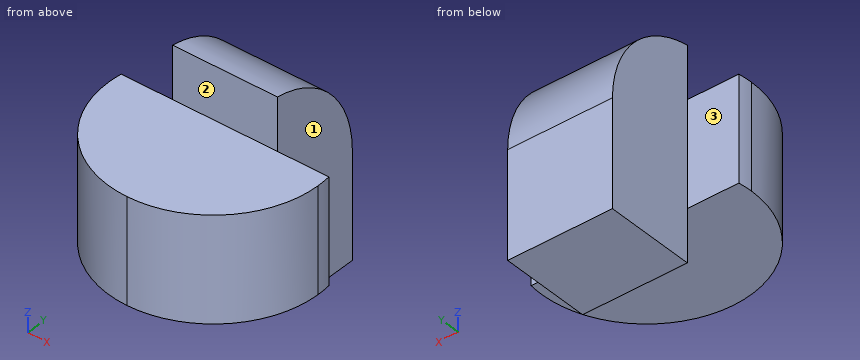
from build123d import *

# Parameters (mm, degrees)
SKETCH1_W           = 40
SKETCH1_H           = 40
BOSS_EXTRUDE1_DEPTH = 40
SKETCH2_W           = 10
SKETCH2_H           = 20
CUT_EXTRUDE1_DEPTH  = 40
SKETCH3_W           = 10
SKETCH3_H           = 10
CUT_EXTRUDE2_DEPTH  = 40
CUT_EXTRUDE3_DEPTH  = 40
SKETCH5_W           = 20
SKETCH5_H           = 10
CUT_EXTRUDE4_DEPTH  = 40
SKETCH6_W           = 20
SKETCH6_H           = 19.641016119
CUT_EXTRUDE5_DEPTH  = 40
BOSS_EXTRUDE2_DEPTH = 20


with BuildPart() as part:
    # Sketch1 → Boss-Extrude1 (new body)
    with BuildSketch(Plane.XY):
        with Locations((20, 20)):
            Rectangle(SKETCH1_W, SKETCH1_H)
    extrude(amount=BOSS_EXTRUDE1_DEPTH)

    # Sketch2 → Cut-Extrude1 (cut)
    with BuildSketch(Plane.XY.offset(40)):
        with BuildLine():
            ThreePointArc((20, 0), (5.857864376, 5.857864376), (0, 20))
            Line((0, 20), (0, 0))
            Line((0, 0), (20, 0))
        make_face()
        with BuildLine():
            ThreePointArc((40, 20), (34.142135624, 5.857864376), (20, 0))
            Line((20, 0), (40, 0))
            Line((40, 0), (40, 20))
        make_face()
        with Locations((35, 30)):
            Rectangle(SKETCH2_W, SKETCH2_H)
        with Locations((5, 30)):
            Rectangle(SKETCH2_W, SKETCH2_H)
    extrude(amount=-CUT_EXTRUDE1_DEPTH, mode=Mode.SUBTRACT)

    # Sketch3 → Cut-Extrude2 (cut)
    with BuildSketch(Plane(origin=(0, 20, 0), x_dir=(1, 0, 0), z_dir=(0, 1, 0))):
        with Locations((5, -5)):
            Rectangle(SKETCH3_W, SKETCH3_H)
        with Locations((35, -5)):
            Rectangle(SKETCH3_W, SKETCH3_H)
        with Locations((35, -35)):
            Rectangle(SKETCH3_W, SKETCH3_H)
        with Locations((5, -35)):
            Rectangle(SKETCH3_W, SKETCH3_H)
    extrude(amount=-CUT_EXTRUDE2_DEPTH, mode=Mode.SUBTRACT)

    # Sketch4 → Cut-Extrude3 (cut)
    with BuildSketch(Plane.ZY.offset(-10)):
        Polygon((10, 22.679491924), (0, 22.679491924), (0, 2.679491924), (10, 2.679491924), (10, 20), align=None)
        Polygon((30, 2.679491924), (40, 2.679491924), (40, 22.679491924), (30, 22.679491924), (30, 20), align=None)
        with BuildLine():
            ThreePointArc((20.358983897, 39.999201827), (33.408185604, 35.000772179), (40, 22.679491924))
            Line((40, 22.679491924), (40, 40))
            Line((40, 40), (20.358983897, 39.999201827))
        make_face()
    extrude(amount=-CUT_EXTRUDE3_DEPTH, mode=Mode.SUBTRACT)

    # Sketch5 → Cut-Extrude4 (cut)
    with BuildSketch(Plane(origin=(0, 2.679491924, 0), x_dir=(1, 0, 0), z_dir=(0, 1, 0))):
        with Locations((20, -5)):
            Rectangle(SKETCH5_W, SKETCH5_H)
        with Locations((20, -35)):
            Rectangle(SKETCH5_W, SKETCH5_H)
    extrude(amount=-CUT_EXTRUDE4_DEPTH, mode=Mode.SUBTRACT)

    # Sketch6 → Cut-Extrude5 (cut)
    with BuildSketch(Plane(origin=(0, 39.998374412, -0.001625456), x_dir=(1, 0, 0), z_dir=(0, -0.999999999, 4.0638e-05))):
        with Locations((20, 30.18111743)):
            Rectangle(SKETCH6_W, SKETCH6_H)
    extrude(amount=-CUT_EXTRUDE5_DEPTH, mode=Mode.SUBTRACT)

    # Sketch8 → Boss-Extrude2 (add)
    with BuildSketch(Plane.XY.offset(30)):
        with BuildLine():
            Line((0.180304669, 22.679491924), (39.819695331, 22.679491924))
            ThreePointArc((39.819695331, 22.679491924), (20, 0), (0.180304669, 22.679491924))
        make_face()
    extrude(amount=-BOSS_EXTRUDE2_DEPTH)


solid = part.part
Could you check a few things on this model? Use its own coordinates, in mm. Face numbers are marked on the shaded views. A direction names the side the tool comes from. Coordinates: 2 decimals unless noted, no trailing zeros. Order: outer loops, then holes, each group sorted by start corner. A loop starts at its lowest first (then second) coordinate and runs counter-clockwise, first axis right, second up. Notation, with made-up numbers: (37, 80) -> (44, 80) arc R18 cw to (44, 99) -> close; hole circle Ø1 at (-18.75, 68.5). An arc over 180 degrees is marked (long way). One line per question, with ' | ' between items.
Q1. I'm going to push flat-ended pins straight in: P1, Ø8.5, axis at y = 29.5, z = 11, coming from the +X side; P2, Ø2, axis at x = 16.5, z = 29, coming from the -Y side; P3, Ø3, axis at x = 25, z = 4, coming from the -Y side; P4, Ø6, axis at x = 4.5, z = 5, coming from the -Y side. Where does each tip first touch, or does it pass through?
Return value:
P1: x = 30 | P2: y = 0.16 | P3: y = 22.68 | P4: through
Q2. Imagine slicing it at C-C on y = 4. Please give me the cut outline in (x, z).
Return value:
outline: (8, 10) -> (32, 10) -> (32, 30) -> (8, 30) -> close
Q3. If I drill on L1, parallel to Z at x = 17, y = 17; L2, parallel to Y at x = 13, z = 9, over which ranges is the centre line in solid material (lowest first)?
Return value:
L1: 10 to 30 | L2: 22.68 to 40
Q4. On a 3-axis mill with a long thin cutter (end or side, diameter ignored), from which of +Z, -Z, +X, -X, +Y, -Y can I reach the whole of each face in a straight line? I mean the marked faces 1, 2 and 3. Say none if no direction works.
Return value:
face 1: +Z, -Z, +X, +Y | face 2: +Z, +X, -X, -Y | face 3: +Z, -Z, -X, +Y
Q5. Imagine slicing it at D-D on z = 8. Please give me the cut outline in (x, y), and give its area (3 significant figures).
Return value:
outline: (10, 22.68) -> (30, 22.68) -> (30, 40) -> (10, 40) -> close | area: 346 mm²
Q6. Imagine slicing it at A-A on z = 16. Please give me the cut outline in (x, y).
Return value:
outline: (0.18, 22.68) arc R20 ccw (long way) to (39.82, 22.68) -> (30, 22.68) -> (30, 40) -> (10, 40) -> (10, 22.68) -> close
